Design review of the part built by this model. Coordinates are the model's own, in mm. Coordinates: 2 decimals unless noted, no trailing zeros. Loops run counter-clockwise (first coordinate to the right, second up) from the corner with the lowest first, then second, coordinate; pieces in that order, holes last. Notation, with made-up numbers: M 39.25,8.5 L 84.25,8.5 A29 cw 84.25,41.5 Z; hole C 34.25,40.5 d7. An arc over 180 degrees is marked long. One line per item, written item: value.
```python
from build123d import *

# Parameters (mm, degrees)
SKETCH3_W           = 125
SKETCH3_H           = 205
BOSS_EXTRUDE1_DEPTH = 3
SKETCH5_W           = 12
SKETCH5_H           = 3
SKETCH5_W_2         = 3
SKETCH5_H_2         = 12
BOSS_EXTRUDE2_DEPTH = 3
SKETCH6_R           = 10
CUT_EXTRUDE1_DEPTH  = 6


with BuildPart() as part:
    # Sketch3 → Boss-Extrude1 (new body)
    with BuildSketch(Plane(origin=(0, 0, 0), x_dir=(1, 0, 0), z_dir=(0, 1, 0))):
        Rectangle(SKETCH3_W, SKETCH3_H)
    extrude(amount=BOSS_EXTRUDE1_DEPTH)

    # Sketch5 → Boss-Extrude2 (add)
    with BuildSketch(Plane(origin=(0, 3, 0), x_dir=(1, 0, 0), z_dir=(0, 1, 0))):
        with Locations((24, -104)):
            Rectangle(SKETCH5_W, SKETCH5_H)
        with Locations((0, -104)):
            Rectangle(SKETCH5_W, SKETCH5_H)
        with Locations((-64, -84)):
            Rectangle(SKETCH5_W_2, SKETCH5_H_2)
        with Locations((-64, -60)):
            Rectangle(SKETCH5_W_2, SKETCH5_H_2)
        with Locations((-64, -12)):
            Rectangle(SKETCH5_W_2, SKETCH5_H_2)
        with Locations((64, -84)):
            Rectangle(SKETCH5_W_2, SKETCH5_H_2)
        with Locations((64, -36)):
            Rectangle(SKETCH5_W_2, SKETCH5_H_2)
        with Locations((64, -12)):
            Rectangle(SKETCH5_W_2, SKETCH5_H_2)
        with Locations((64, 12)):
            Rectangle(SKETCH5_W_2, SKETCH5_H_2)
        with Locations((64, 36)):
            Rectangle(SKETCH5_W_2, SKETCH5_H_2)
        with Locations((64, 84)):
            Rectangle(SKETCH5_W_2, SKETCH5_H_2)
        with Locations((24, 104)):
            Rectangle(SKETCH5_W, SKETCH5_H)
        with Locations((0, 104)):
            Rectangle(SKETCH5_W, SKETCH5_H)
        with Locations((-24, 104)):
            Rectangle(SKETCH5_W, SKETCH5_H)
        with Locations((-48, 104)):
            Rectangle(SKETCH5_W, SKETCH5_H)
        with Locations((-64, 36)):
            Rectangle(SKETCH5_W_2, SKETCH5_H_2)
        with Locations((-64, 12)):
            Rectangle(SKETCH5_W_2, SKETCH5_H_2)
        with Locations((48, -104)):
            Rectangle(SKETCH5_W, SKETCH5_H)
        with Locations((-24, -104)):
            Rectangle(SKETCH5_W, SKETCH5_H)
        with Locations((-48, -104)):
            Rectangle(SKETCH5_W, SKETCH5_H)
        with Locations((-64, -36)):
            Rectangle(SKETCH5_W_2, SKETCH5_H_2)
        with Locations((64, -60)):
            Rectangle(SKETCH5_W_2, SKETCH5_H_2)
        with Locations((64, 60)):
            Rectangle(SKETCH5_W_2, SKETCH5_H_2)
        with Locations((48, 104)):
            Rectangle(SKETCH5_W, SKETCH5_H)
        with Locations((-64, 84)):
            Rectangle(SKETCH5_W_2, SKETCH5_H_2)
        with Locations((-64, 60)):
            Rectangle(SKETCH5_W_2, SKETCH5_H_2)
    extrude(amount=-BOSS_EXTRUDE2_DEPTH)

    # Sketch6 → Cut-Extrude1 (cut)
    with BuildSketch(Plane(origin=(0, 3, 0), x_dir=(1, 0, 0), z_dir=(0, 1, 0))):
        with Locations((22.817541634, -45.5)):
            Circle(SKETCH6_R)
    extrude(amount=-CUT_EXTRUDE1_DEPTH, mode=Mode.SUBTRACT)


solid = part.part
```
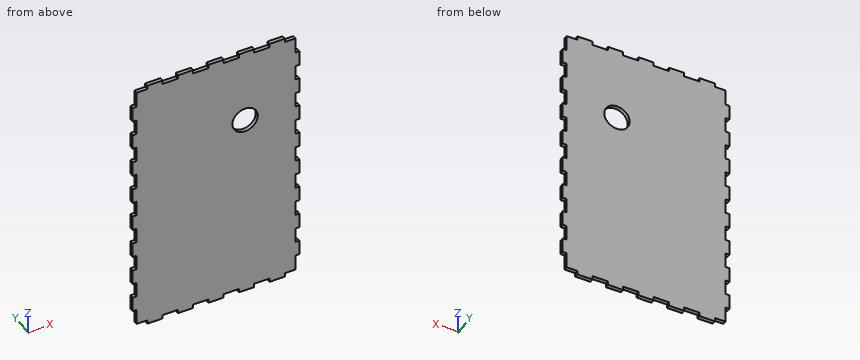
(1) We need section B-B on z = 92. State the section outline as (x, y) points, then the cut area to 3 significant figures.
Reply:
outline: M -62.5,0 L 62.5,0 L 62.5,3 L -62.5,3 Z
area: 375 mm2
(2) To check wall thickness, follow line 1 along X through (y, z) = (1.05, 45.5); line 2 along Z through (x, y) = (22.5, 1.15); line 3 along Z through (x, y) = (10, 2.4). State the ranges of each line that lie inside material, in increasing order. Write a range as [from, to].
Reply:
line 1: x = [-62.5, 12.82], [32.82, 62.5]
line 2: z = [-105.5, 35.51], [55.49, 105.5]
line 3: z = [-102.5, 102.5]
(3) Insertion check: pin 1 (1 mm diameter, centred on x = 33, y = 2.5, fed in from +Z); pin 2 (0.9 mm diameter, centred on y = 1, z = 103.5, fed in from -X); pin 3 (1.5 mm diameter, centred on y = 1, z = 104, fed in from +X). Each pin has a flat end and moves straight along its axis. Give the tip position at first contact, or say it passes through.
Reply:
pin 1: stops at z = 102.5
pin 2: stops at x = -54
pin 3: stops at x = 54
(4) We need section A-A on z = 45.5. State the section outline as (x, y) points.
Reply:
outline: M -62.5,0 L 12.82,0 L 12.82,3 L -62.5,3 Z; M 32.82,0 L 62.5,0 L 62.5,3 L 32.82,3 Z
(5) We need section C-C on x = 8. State the section outline as (y, z) points.
Reply:
outline: M 0,-102.5 L 3,-102.5 L 3,102.5 L 0,102.5 Z
